Here's how the part is built. I have some questions about the finished solid (model axes, mm). Face numbers are marked on the shaded views. A direction names the side the tool comes from. Round coordinates to 2 decimals unless told otherwise and drop trailing zeros. Loops run counter-clockwise (first coordinate to the right, second up) from the corner with the lowest first, then second, coordinate; pieces in that order, holes last. Notation, with made-up numbers: M 82.5,-39.5 L 114.5,-39.5 A22 cw 114.5,-28.5 Z; hole C -28,19.25 d3. An arc over 180 degrees is marked long. Answer as a JSON object with one key per item and string values.
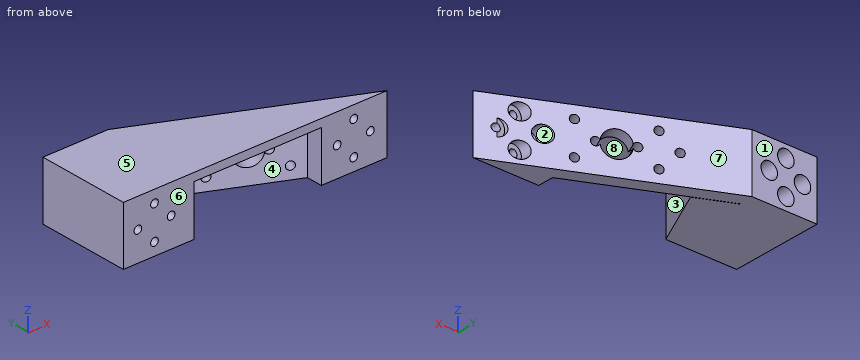
Autodesk Inventor part; units mm, degrees
ref_plane "Work Plane11" through (0, 3.81, 0) normal (0, -1, 0) x (1, 0, 0)
ref_plane "Work Plane12" through (28.6903, 38.8361, 27.94) normal (0.4226, 0.9063, 0) x (0.9063, -0.4226, 0)
ref_plane "YZ Plane" through (0, 0, 0) normal (1, 0, 0) x (0, 1, 0)
sketch "Sketch17" plane through (0, 0, 0) normal (0, 0, 1) x (1, 0, 0)
  line L0 (0, 0) -> (127, 0)
  line L1 (127, 0) -> (31.3739, 44.5912)
  line L2 (0, 44.5912) -> (0, 0)
  line L3 (0, 44.5912) -> (31.3739, 44.5912)
  dimension "d78" = 127
  dimension "d79" = 25
extrude "Extrusion20" add sketch "Sketch17" along normal blind 25.4
sketch "Sketch18" plane through (0, 0, 0) normal (0, -1, 0) x (1, 0, 0)
  line L0 (127.0002, 25.3999) -> (0.1269, 25.3999)
  line L1 (0.1269, 25.3999) -> (0.1269, -0.0001)
  line L2 (127.0002, -0.0001) -> (0.1269, -0.0001)
  line L3 (127.0002, 25.3999) -> (127.0002, -0.0001)
  circle A0 centre (111.0002, 22) radius 1.85
  circle A1 centre (111.0002, 6) radius 1.85
  circle A2 centre (119.0002, 14) radius 1.85
  circle A3 centre (103.0002, 14) radius 1.85
  circle A4 centre (7.0002, 14) radius 1.85
  circle A5 centre (15.0002, 22) radius 1.85
  circle A6 centre (15.0002, 6) radius 1.85
  circle A7 centre (23.0002, 14) radius 1.85
  point P0 (0, 0)
  point P1 (50.8002, 25.3999)
sketch "Sketch19" plane through (0, 0, 25.4) normal (0, 0, 1) x (1, 0, 0)
  line L0 (0, 0) -> (127, 0)
  line L1 (127, 0) -> (31.3739, 44.5912)
  line L2 (31.3739, 44.5912) -> (0, 44.5912)
  line L3 (0, 44.5912) -> (0, 0)
extrude "Extrusion21" add sketch "Sketch19" along normal blind 2.54
extrude "Extrusion22" cut sketch "Sketch18" against normal up to next contours A0 | A1 | A2 | A3 | A4 | A5 | A6 | A7
ref_plane "Work Plane11" through (0, 3.81, 0) normal (0, -1, 0) x (1, 0, 0)
sketch "Sketch20" plane through (0, 3.81, 0) normal (0, -1, 0) x (1, 0, 0)
  circle A0 centre (15.0002, 22) radius 1.85
  circle A1 centre (15.0002, 22) radius 3.9751
  circle A2 centre (7.0002, 14) radius 1.85
  circle A3 centre (7.0002, 14) radius 3.9751
  circle A4 centre (15.0002, 6) radius 1.85
  circle A5 centre (15.0002, 6) radius 3.9751
  circle A6 centre (23.0002, 14) radius 1.85
  circle A7 centre (23.0002, 14) radius 3.9751
  circle A8 centre (103.0002, 14) radius 1.85
  circle A9 centre (103.0002, 14) radius 3.9751
  circle A10 centre (111.0002, 22) radius 1.85
  circle A11 centre (111.0002, 22) radius 3.9751
  circle A12 centre (111.0002, 6) radius 1.85
  circle A13 centre (111.0002, 6) radius 3.9751
  circle A14 centre (119.0002, 14) radius 1.85
  circle A15 centre (119.0002, 14) radius 3.9751
  point P0 (0, 0)
  dimension "d100" = 7.9502
  dimension "d101" = 7.9502
  dimension "d102" = 7.9502
  dimension "d103" = 7.9502
  dimension "d104" = 7.9502
  dimension "d105" = 7.9502
  dimension "d106" = 7.9502
  dimension "d107" = 7.9502
extrude "Extrusion23" cut sketch "Sketch20" against normal up to next
ref_plane "Work Plane12" through (28.6903, 38.8361, 27.94) normal (0.4226, 0.9063, 0) x (0.9063, -0.4226, 0)
sketch "Sketch21" plane through (0, 0, 0) normal (0, -1, 0) x (1, 0, 0)
  line L0 (30.6202, 24.13) -> (95.3802, 24.13)
  line L1 (95.3802, 24.13) -> (95.3802, 0)
  line L2 (95.3802, 0) -> (30.6202, 0)
  line L3 (30.6202, 0) -> (30.6202, 24.13)
  line L4 (0, 27.94) -> (127, 27.94) construction
  line L5 (0, 0) -> (127, 0) construction
  circle A0 centre (23.0002, 14) radius 1.85 construction
  circle A1 centre (103.0002, 14) radius 1.85 construction
  dimension "d112" = 3.81
  dimension "d113" = 0
  dimension "d114" = 7.62
  dimension "d115" = 7.62
extrude "Extrusion24" cut sketch "Sketch21" against normal up to surface surface through (28.6903, 38.8361, 27.94) normal (0.4226, 0.9063, 0)
sketch "Sketch23" plane through (0, 0, 27.94) normal (0, 0, 1) x (1, 0, 0)
  line L0 (0, 0) -> (127, 0) construction
  line L1 (127, 0) -> (50.8, 0) construction
  line L2 (50.8, 0) -> (50.8, 35.5326) construction
  line L3 (127, 0) -> (31.3739, 44.5912) construction
  dimension "d119" = 76.2
sketch "Sketch24" plane through (31.3739, 44.5912, 27.94) normal (0.4226, 0.9063, 0) x (0.9063, -0.4226, 0)
  circle A0 centre (35.1489, 5.94) radius 1.85
  circle A1 centre (27.1489, 13.94) radius 1.85
  circle A2 centre (35.1489, 21.94) radius 1.85
  circle A3 centre (43.1489, 13.94) radius 1.85
  circle A4 centre (51.1489, 13.94) radius 4
  circle A5 centre (59.1489, 13.94) radius 1.85
  circle A6 centre (67.1489, 5.94) radius 1.85
  circle A7 centre (75.1489, 13.94) radius 1.85
  circle A8 centre (67.1489, 21.94) radius 1.85
  circle A9 centre (51.1489, 13.94) radius 6.35
  circle A10 centre (67.1489, 5.94) radius 1.9542
  circle A11 centre (75.1489, 13.94) radius 3.9195
  circle A12 centre (67.1489, 21.94) radius 1.9542
  circle A13 centre (59.1489, 13.94) radius 1.9542
  circle A14 centre (43.1489, 13.94) radius 1.9542
  circle A15 centre (35.1489, 5.94) radius 1.9542
  circle A16 centre (27.1489, 13.94) radius 1.9542
  circle A17 centre (35.1489, 21.94) radius 1.9542
  point P0 (-9.5894, 27.94)
  dimension "d120" = 12.7
  dimension "d125" = 3.9084
  dimension "d126" = 3.9084
  dimension "d127" = 3.9084
  dimension "d128" = 3.9084
  dimension "d129" = 3.9084
  dimension "d130" = 3.9084
  dimension "d131" = 3.9084
extrude "Extrusion25" cut sketch "Sketch24" against normal up to surface (6.35 mm away) contours A0 | A1 | A2 | A3 A9 | A3 A9 A14 | A9 A3 | A3 A9 A14 | A9 A13 A14 | A13 A9 A5 | A9 A5 A13 | A9 A5 | A5 A9 | A4 | A6 | A8 | A10 | A12 | A15 | A16 | A17
sketch "Sketch27" plane through (95.3802, 0, 24.13) normal (0, 0, -1) x (-1, 0, 0)
  line L0 (64.76, 0) -> (0, 0)
  line L1 (64.76, 0) -> (64.76, 37.7416)
  line L2 (64.76, 37.7416) -> (47.4149, 29.6534)
  line L3 (43.8558, 28.1884) -> (40.3136, 26.5366)
  line L4 (47.4149, 29.6534) -> (61.2425, 0)
  line L5 (61.2425, 0) -> (64.76, 0)
  point P0 (95.3802, 0)
extrude "Extrusion27" add sketch "Sketch27" along normal up to surface (24.13 mm away)
properties part number "IntakeCchannelMount"
Item 1: For the marked faces 1, 2, 3, 4 and 5, which set-ups out of +Z, -Z, +X, -X, +Y, -Y let a thin tool reach every point of the face, with its end or its side?
Solution:
{"face 1": "+Z, -Z, +X, -X, +Y", "face 2": "+Y", "face 3": "-Z, -Y", "face 4": "-Z", "face 5": "+Z, +X, -X, +Y, -Y"}
Item 2: I want a section at B-B on y = 36.5. List the corners of the cut face in (x, z) for me.
Solution:
{"outline": "M 0,0 L 33.28,0 L 33.28,24.13 L 33.7,24.13 L 33.7,0 L 48.73,0 L 48.73,27.94 L 0,27.94 Z; hole C 7,14 d7.95; hole C 15,6 d7.95; hole C 15,22 d7.95; hole C 23,14 d7.95"}
Item 3: I want a section at A-A on z = 6. Count the separate pieces of the cut face and the enclosed holes in it, plus the area to 3 significant figures.
Solution:
{"separate pieces": "5", "enclosed holes": "0", "area": "2,000 mm2"}
Item 4: For P1, Ø8.5, axis at x = 102, z = 14, coming from the +Y side; P2, Ø2, axis at x = 108.5, z = 17.5, coming from the +Y side; P3, Ø4, axis at x = 112, z = 22, coming from the +Y side; P4, Ø3.5, axis at x = 15, z = 6, coming from the -Y side, each with a flat end and sliding along its axis, tell me the tip position at first contact or that it passes through.
Solution:
{"P1": "stops at y = 13.64", "P2": "stops at y = 9.09", "P3": "stops at y = 3.81", "P4": "passes through"}
Item 5: We'd pull the mould along X, two halves only. Please class the marked faces 6, 7 and 8: +X half, -X half, draft (parallel to the pull), parting line (faces both ways), or undercut.
Solution:
{"face 6": "draft", "face 7": "+X half", "face 8": "undercut"}
Item 6: If I drill on L1, parallel to Z at x = 15, y = 9; L2, parallel to X at y = 25, z = 14.25; L3, parallel to X at y = 22.5, z = 13.5, over which ranges is the centre line in solid material (lowest first)? Write a range as from..to.
Solution:
{"L1": "z = 0..2.02, 9.98..18.02, 25.98..27.94", "L2": "x = 0..3.03, 10.97..19.03, 26.97..45.8, 58.36..67.71", "L3": "x = 0..3.06, 10.94..19.06, 26.94..44.63, 63.72..66.6"}
